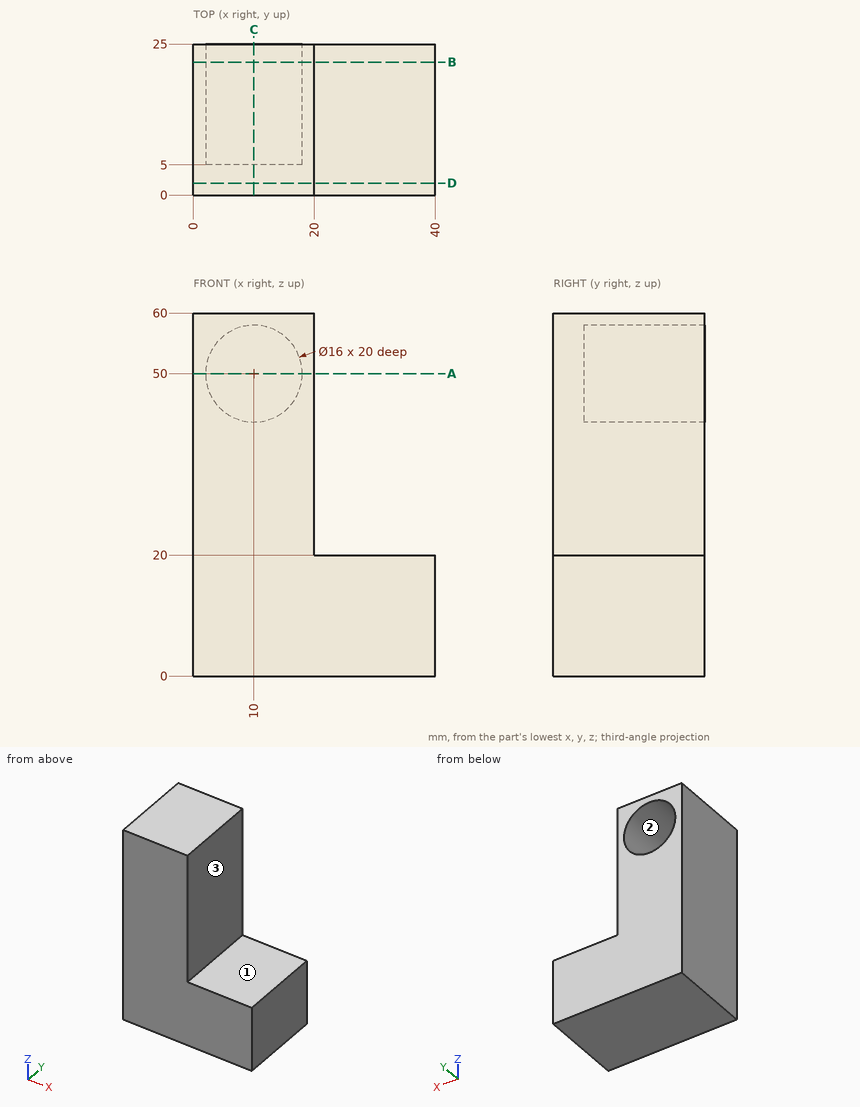
Geometry check sheet. Reference: drawing and pictorial views, mm from the part's lowest x, y, z. Give positions to 0.01 mm unless a question says otherwise; leave off trailing zeros. Write each loop counter-clockwise with the first axis right and the second up, starting at its lowest first coordinate (ties: lowest second). Pieces come first, ordered by that corner, then holes. Notation, with made-up numbers: M 27,21 L 48,21 A20 cw 48,29 Z; hole C -10,-21 d7. An arc over 180 degrees is marked long. Put each result on its own line as item: value. Start each with the question number.
1. Section check A-A (z = 50). Record the cut outline in (x, y), and give its area (3 significant figures).
2. Go/stop test with flat-tipped pins: pin 1 Ø12.5 at (y, z) = (16, 48) entering from +X; pin 2 Ø13 at (x, z) = (9.5, 50.5) entering from +Y; pin 3 Ø6 at (x, y) = (31.5, 17) entering from +Z. Record where each tip stops, or that it passes through.
3. Scan lines: line 1 along Z through (x, y) = (10, 11.75); line 2 along Z through (x, y) = (8.5, 5.75); line 3 along X through (y, z) = (7.5, 29.5). Record each from-to range of solid material in increasing order. Write a range as [from, to].
4. Section check D-D (y = 2). Record the cut outline in (x, z), and give its area (3 significant figures).
5. Section check C-C (x = 10). Record the cut outline in (y, z).
6. Section check B-B (y = 22). Record the cut outline in (x, z).
7. Draft check along Z on the marked faces 1, 2 and 3. Enter one of: +Z half, -Z half, draft (parallel to the pull), parting line (faces both ways), or undercut.
Answer list:
1. outline: M 0,0 L 20,0 L 20,25 L 18,25 L 18,5 L 2,5 L 2,25 L 0,25 Z
1. area: 180 mm2
2. pin 1: x = 20
2. pin 2: y = 5
2. pin 3: z = 20
3. line 1: [0, 42], [58, 60]
3. line 2: [0, 42.14], [57.86, 60]
3. line 3: [0, 20]
4. outline: M 0,0 L 40,0 L 40,20 L 20,20 L 20,60 L 0,60 Z
4. area: 1,600 mm2
5. outline: M 0,0 L 25,0 L 25,42 L 5,42 L 5,58 L 25,58 L 25,60 L 0,60 Z
6. outline: M 0,0 L 40,0 L 40,20 L 20,20 L 20,60 L 0,60 Z; hole C 10,50 d16
7. face 1: +Z half
7. face 2: undercut
7. face 3: draft
